```python
from build123d import *

# Parameters (mm, degrees)
F1_DEPTH = 20
F2_R     = 5
F3_DEPTH = 20.001
F4_R     = 5
F5_R     = 5
F6_R     = 2.5
F7_DEPTH = 23.001


with BuildPart() as f1:
    # F0 (on Right) → F1 (new body)
    with BuildSketch(Plane.YZ):
        Polygon((-27.5, -10), (-27.5, -13), (27.5, -13), (27.5, -10), (10, -10), (10, 10), (-10, 10), (-10, -10), align=None)
    extrude(amount=F1_DEPTH)

    # F2 (on face) → F3 (cut, through all)
    with BuildSketch(Plane.YZ.offset(20)):
        Circle(F2_R)
    extrude(amount=-F3_DEPTH, mode=Mode.SUBTRACT)

    # F4
    f4_edges = [f1.edges().sort_by_distance(p)[0] for p in [
        (10, -10, 10),
    ]]
    fillet(f4_edges, radius=F4_R)

    # F5
    f5_edges = [f1.edges().sort_by_distance(p)[0] for p in [
        (10, 10, 10),
    ]]
    fillet(f5_edges, radius=F5_R)

    # F6 (on face) → F7 (cut, through all)
    with BuildSketch(Plane(origin=(0, 0, -13), x_dir=(1, 0, 0), z_dir=(0, 0, -1))):
        with Locations((10, 17.5)):
            Circle(F6_R)
        with Locations((10, -17.5)):
            Circle(F6_R)
    extrude(amount=-F7_DEPTH, mode=Mode.SUBTRACT)


solid = f1.part
```
The model under review builds one solid part; all positions refer to its coordinate system, in mm. A direction names the side the tool comes from. Round coordinates to 2 decimals unless told otherwise and drop trailing zeros. Loops run counter-clockwise (first coordinate to the right, second up) from the corner with the lowest first, then second, coordinate; pieces in that order, holes last. Notation, with made-up numbers: M -16.75,56.5 L 19.25,56.5 A24 ccw 19.25,94.5 Z; hole C 80,16 d9. An arc over 180 degrees is marked long. Put each result on its own line as item: value.
Q1. For pin 1 (7.5 mm diameter, centred on x = 7.5, z = -5.5, fed in from +Y); pin 2 (5 mm diameter, centred on x = 6, y = -21.5, fed in from +Z); pin 3 (12 mm diameter, centred on y = 16, z = 7, fed in from -X), all flat-tipped, find the tip position at first contact; note any pin that passes through.
Result set:
pin 1: stops at y = 10
pin 2: stops at z = -10
pin 3: passes through
Q2. Consider section D-D, the plane x = 17.25. Give the boundary of the cut face in (y, z), then the cut area to 3 significant figures.
Result set:
outline: M -27.5,-13 L 27.5,-13 L 27.5,-10 L 10,-10 L 10,5 A5 ccw 5,10 L -5,10 A5 ccw -10,5 L -10,-10 L -27.5,-10 Z; hole C 0,0 d10
area: 476 mm²
Q3. Consider section A-A, the plane x = 10. Give the boundary of the cut face in (y, z).
Result set:
outline: M -27.5,-13 L -20,-13 L -20,-10 L -27.5,-10 Z; M -15,-13 L 15,-13 L 15,-10 L 10,-10 L 10,5 A5 ccw 5,10 L -5,10 A5 ccw -10,5 L -10,-10 L -15,-10 Z; M 20,-13 L 27.5,-13 L 27.5,-10 L 20,-10 Z; hole C 0,0 d10
Q4. Consider section C-C, the plane z = 0. Give the boundary of the cut face in (x, y), then the cut area to 3 significant figures.
Result set:
outline: M 0,-10 L 20,-10 L 20,-5 L 0,-5 Z; M 0,5 L 20,5 L 20,10 L 0,10 Z
area: 200 mm²
Q5. Mouldability with a two-part tool opening along Y and no side actions: class faces 1 (the cylindrical face through (10, -20, -12)), 2 (the flat face through (10, 27.5, -12)), 3 (the flat face through (20, 2, -5)), 4 (the cylindrical face through (10, -9, 8)) as released by +Y, released by -Y, zero draft, split by the parting line, or undercut.
Result set:
face 1: undercut
face 2: released by +Y
face 3: zero draft
face 4: released by -Y
Q6. Machinability: for faces 5 (the flat face through (10, -21, -10)), 6 (the cylindrical face through (10.14, -1.08, -4.88)), 7 (the flat face through (10, 10, -3)), which of the approach directions +Z, -Z, +X, -X, +Y, -Y give a long, thin tool a straight path to every point of the face, cutting with its end or side? Answer none if there is none.
Result set:
face 5: +Z, +X, -X, -Y
face 6: +X, -X
face 7: +Z, +X, -X, +Y
Q7. To check wall thickness, follow L1, parallel to Y at x = 10, z = -11.2; L2, parallel to X at y = -17.5, z = -10.9; L3, parallel to Z at x = 9.25, y = 0. State the ranges of each line that lie inside material, in increasing order.
Result set:
L1: y = -27.5 to -20, -15 to 15, 20 to 27.5
L2: x = 0 to 7.5, 12.5 to 20
L3: z = -13 to -5, 5 to 10
Q8. Consider section B-B, the plane y = 0. Give the boundary of the cut face in (x, z), then the cut area to 3 significant figures.
Result set:
outline: M 0,-13 L 20,-13 L 20,-5 L 0,-5 Z; M 0,5 L 20,5 L 20,10 L 0,10 Z
area: 260 mm²
